from build123d import *

# Parameters (mm, degrees)
SKETCH_1_R      = 1
SKETCH_1_R_2    = 1.5
EXTRUDE_1_DEPTH = 3


with BuildPart() as part:
    # 스케치1 → 보스-돌출1 (new body)
    with BuildSketch(Plane.XY):
        with BuildLine():
            Line((-2.794, 4), (0, 4))
            ThreePointArc((0, 4), (4, 0), (0, -4))
            Line((0, -4), (-2.794, -4))
            ThreePointArc((-2.794, -4), (-6.794, 0), (-2.794, 4))
        make_face()
        with Locations((-2.794, 0)):
            Circle(SKETCH_1_R, mode=Mode.SUBTRACT)
        Circle(SKETCH_1_R_2, mode=Mode.SUBTRACT)
    extrude(amount=EXTRUDE_1_DEPTH)


solid = part.part
For this review, take the finished solid that the model builds, in its own axes (mm). Round coordinates to 2 decimals unless told otherwise and drop trailing zeros. Order: outer loops, then holes, each group sorted by start corner. A loop starts at its lowest first (then second) coordinate and runs counter-clockwise, first axis right, second up. Notation, with made-up numbers: M 41.25,-36.75 L 60.25,-36.75 A7 ccw 60.25,-29.75 Z; hole C -12,53 d4. An arc over 180 degrees is marked long. Use a Markdown table: item, result. Add a question column.
Item 1: Add section D-D, the plane y = 1.25. Give the boundary of the cut face in (x, z).
Item 2: Add section A-A, the plane y = 0. Give the boundary of the cut face in (x, z), then the cut area to 3 significant figures.
Item 3: Mouldability with a two-part tool opening along Y and no side actions: class faces 1 (the flat face through (-1, 2, 0)), 2 (the flat face through (-1, -4, 1)), 3 (the cylindrical face through (-1.5, 0.07, 1.48)) as released by +Y, released by -Y, zero draft, split by the parting line, or undercut.
Item 4: Insertion check: pin 1 (1 mm diameter, centred on y = -1.5, z = 2.5, fed in from +X). The pin has a flat end and moves straight along its axis. Give the tip position at first contact, or say it passes through.
Item 5: Add section B-B, the plane z = 0.6. Give the boundary of the cut face in (x, y), then the cut area to 3 significant figures.
Item 6: Add section C-C, the plane x = 0.5. Give the boundary of the cut face in (y, z), then the cut area to 3 significant figures.
Item 7: To check wall thickness, follow line 1 along X through (y, z) = (0.75, 1.25); line 2 along Y through (x, z) = (-2.75, 2.25); line 3 along Y through (x, z) = (-0.75, 0.95). State the ranges of each line that lie inside material, in increasing order.
Geometry results:
| question | item | result |
|---|---|---|
| 1 | outline | M -6.59,0 L -0.83,0 L -0.83,3 L -6.59,3 Z; M 0.83,0 L 3.8,0 L 3.8,3 L 0.83,3 Z |
| 2 | outline | M -6.79,0 L -3.79,0 L -3.79,3 L -6.79,3 Z; M -1.79,0 L -1.5,0 L -1.5,3 L -1.79,3 Z; M 1.5,0 L 4,0 L 4,3 L 1.5,3 Z |
| 2 | area | 17.4 mm² |
| 3 | face 1 | zero draft |
| 3 | face 2 | released by -Y |
| 3 | face 3 | undercut |
| 4 | pin 1 | stops at x = 3.87 |
| 5 | outline | M -2.79,-4 L 0,-4 A4 ccw 0,4 L -2.79,4 A4 ccw Z; hole C -2.79,0 d2; hole C 0,0 d3 |
| 5 | area | 62.4 mm² |
| 6 | outline | M -3.97,0 L -1.41,0 L -1.41,3 L -3.97,3 Z; M 1.41,0 L 3.97,0 L 3.97,3 L 1.41,3 Z |
| 6 | area | 15.3 mm² |
| 7 | line 1 | x = -6.72 to -3.46, -2.13 to -1.3, 1.3 to 3.93 |
| 7 | line 2 | y = -4 to -1, 1 to 4 |
| 7 | line 3 | y = -4 to -1.3, 1.3 to 4 |
